```python
from build123d import *

# Parameters (mm, degrees)
SKETCH_4_R          = 6.85
SKETCH_4_R_2        = 2.15
CUT_EXTRUDE_1_DEPTH = 51.079936266
SKETCH_6_R          = 21.3
SKETCH_6_R_2        = 12.1
CUT_EXTRUDE_3_DEPTH = 3.3
SKETCH_7_R          = 7.85
CUT_EXTRUDE_4_DEPTH = 10


with BuildPart() as part:
    # 草图3 → 放样1 section 0
    with BuildSketch(Plane(origin=(0, 14, 0), x_dir=(1, 0, 0), z_dir=(0, 1, 0))):
        with BuildLine():
            Line((25, 10.355339059), (10.355339059, 25))
            Line((10.355339059, 25), (-10.355339059, 25))
            Line((-10.355339059, 25), (-25, 10.355339059))
            Line((-25, 10.355339059), (-25, -10.355339059))
            Line((-25, -10.355339059), (-10.355339059, -25))
            Line((-10.355339059, -25), (10.355339059, -25))
            Line((10.355339059, -25), (25, -10.355339059))
            Line((25, -10.355339059), (25, 10.355339059))
        make_face()
    # 草图1 → 放样1 section 1
    with BuildSketch(Plane(origin=(0, 0, 0), x_dir=(1, 0, 0), z_dir=(0, 1, 0))):
        with BuildLine():
            Line((34, -14.083261121), (34, 14.083261121))
            Line((34, 14.083261121), (14.083261121, 34))
            Line((14.083261121, 34), (-14.083261121, 34))
            Line((-14.083261121, 34), (-34, 14.083261121))
            Line((-34, 14.083261121), (-34, -14.083261121))
            Line((-34, -14.083261121), (-14.083261121, -34))
            Line((-14.083261121, -34), (14.083261121, -34))
            Line((14.083261121, -34), (34, -14.083261121))
        make_face()
    loft()

    # 草图4 → 切除-拉伸1 (cut, through all)
    with BuildSketch(Plane(origin=(0, 14, 0), x_dir=(1, 0, 0), z_dir=(0, 1, 0))):
        with Locations(Location((0, 0, 0), (0, 0, 270))):
            Circle(SKETCH_4_R)
        with Locations(Location((-29.157457896, 12.077414505, 0), (0, 0, 270))):
            Circle(SKETCH_4_R_2)
        with Locations(Location((29.157457896, 12.077414505, 0), (0, 0, 270))):
            Circle(SKETCH_4_R_2)
        with Locations(Location((29.157457896, -12.077414505, 0), (0, 0, 270))):
            Circle(SKETCH_4_R_2)
        with Locations(Location((12.077414505, -29.157457896, 0), (0, 0, 270))):
            Circle(SKETCH_4_R_2)
        with Locations(Location((-12.077414505, -29.157457896, 0), (0, 0, 270))):
            Circle(SKETCH_4_R_2)
        with Locations(Location((-29.157457896, -12.077414505, 0), (0, 0, 270))):
            Circle(SKETCH_4_R_2)
    extrude(amount=-CUT_EXTRUDE_1_DEPTH, mode=Mode.SUBTRACT)

    # 草图6 → 切除-拉伸3 (cut)
    with BuildSketch(Plane(origin=(0, 14, 0), x_dir=(1, 0, 0), z_dir=(0, 1, 0))):
        with Locations(Location((0, 0, 0), (0, 0, 270))):
            Circle(SKETCH_6_R)
        with Locations(Location((0, 0, 0), (0, 0, 270))):
            Circle(SKETCH_6_R_2, mode=Mode.SUBTRACT)
    extrude(amount=-CUT_EXTRUDE_3_DEPTH, mode=Mode.SUBTRACT)

    # 草图7 → 切除-拉伸4 (cut)
    with BuildSketch(Plane.XZ):
        with Locations(Location((0, 0, 0), (0, 0, 270))):
            Circle(SKETCH_7_R)
    extrude(amount=-CUT_EXTRUDE_4_DEPTH, mode=Mode.SUBTRACT)


solid = part.part
```
Geometry check sheet. Reference: the model listing, model coordinates, mm. A direction names the side the tool comes from. Coordinates: 2 decimals unless noted, no trailing zeros. Answer in a Markdown table with one row per item. Add a question column.
1. Section check A-A (y = 2.25). Give the number of separate pieces and of enclosed holes in the cut face, plus the area to 3 significant figures.
2. Material ranges on L1, parallel to X at y = 11.5, z = 7.5; L2, parallel to Y at x = -10.5, z = -11; L3, parallel to Z at x = 29, y = 7.5, recorded low to high. Write a range as [from, to].
3. Access from +Z, -Z, +X, -X, +Y, -Y to the whole of each face (thin tool, end or side, straight path). Record for faces 3 (the face through (17.96, 12.37, 11.45)), 4 (the face through (-4.777, 4.93, 6.229)), 5 (the face through (-11.98, 4.21, 27.01)).
4. Gauge pin test, flat ends, axial feed: pin 1 Ø4 at (x, z) = (29.16, -12.08) entering from +Y; pin 2 Ø5 at (x, y) = (10, 7) entering from +Z; pin 3 Ø8 at (x, y) = (5.5, 10) entering from -Z; pin 4 Ø12 at (x, z) = (21.5, 24.5) entering from +Y. Record the tip position at first contact, or that the pin passes through.
5. Draft check along X on faces 1 (the face through (10, 14, -19)), 2 (the face through (-9, 10.7, 9)). Enter one of: +X half, -X half, draft (parallel to the pull), parting line (faces both ways), or undercut.
Data:
| question | item | result |
|---|---|---|
| 1 | separate pieces | 1 |
| 1 | enclosed holes | 7 |
| 1 | area | 3,230 mm² |
| 2 | L1 | x = [-26.61, -19.94], [-9.5, 9.5], [19.94, 26.61] |
| 2 | L2 | y = [0, 10.7] |
| 2 | L3 | z = [-9.93, 9.93] |
| 3 | face 3 | +Y |
| 3 | face 4 | -Y |
| 3 | face 5 | +Y, -Y |
| 4 | pin 1 | passes through |
| 4 | pin 2 | stops at z = 31.11 |
| 4 | pin 3 | stops at z = -30.14 |
| 4 | pin 4 | stops at y = 11.62 |
| 5 | face 1 | draft |
| 5 | face 2 | undercut |
